Design review of the part built by this model. Coordinates are the model's own, in mm. Round coordinates to 2 decimals unless told otherwise and drop trailing zeros. Order: outer loops, then holes, each group sorted by start corner. A loop starts at its lowest first (then second) coordinate and runs counter-clockwise, first axis right, second up. Notation, with made-up numbers: M 70,-11 L 115,-11 A24 cw 115,24 Z; hole C 54,15 d3. An arc over 180 degrees is marked long. Use a Markdown table: item, result. Add a question column.
(1) The part is to be moulded in two halves that separate along Z. For faces 1 (the face through (434.95, 2.03, -85.78)), 2 (the face through (222, 4, -127)), say which applies: released by +Z, released by -Z, zero draft, split by the parting line, or undercut.
(2) To check wall thickness, follow probe 1 along X at (y, z) = (1.4, -190); probe 2 along X at (y, z) = (3.6, -114.5); probe 3 along X at (y, z) = (2.45, -197.5). State the ranges of each line that lie inside material, in increasing order. Write a range as from..to.
(3) Take a section at D-D (z = -211.5). Write out the cut boundary in (x, y).
(4) Take a section at B-B (z = -65). Write out the cut boundary in (x, y), then the cut area to 3 significant figures.
(5) Take a section at C-C (x = 429). Write out the cut boundary in (y, z).
(6) For pin 1 (0.6 mm diameter, centred on y = 2, z = -114.5, fed in from -X); pin 2 (7 mm diameter, centred on x = 429, z = -65, fed in from -Y), all flat-tipped, find the tip position at first contact; note any pin that passes through.
(7) Take a section at A-A (x = 363). Write out the cut boundary in (y, z).
```python
from build123d import *

# Parameters (mm, degrees)
SKETCH_1_W          = 450
SKETCH_1_H          = 250
EXTRUDE_1_DEPTH     = 4
SKETCH_2_R          = 30
CUT_EXTRUDE_1_DEPTH = 515.797047389
SKETCH_3_R          = 6
SKETCH_3_W          = 20
SKETCH_3_H          = 2
CUT_EXTRUDE_2_DEPTH = 515.797047389


with BuildPart() as part:
    # 草圖1 → 填料-伸長1 (new body)
    with BuildSketch(Plane(origin=(0, 0, 0), x_dir=(1, 0, 0), z_dir=(0, 1, 0))):
        with Locations((225, 125)):
            Rectangle(SKETCH_1_W, SKETCH_1_H)
    extrude(amount=EXTRUDE_1_DEPTH)

    # 草圖2 → 除料-伸長1 (cut, through all)
    with BuildSketch(Plane(origin=(0, 4, 0), x_dir=(1, 0, 0), z_dir=(0, 1, 0))):
        with Locations(Location((78, 190, 0), (0, 0, 270))):
            Circle(SKETCH_2_R)
        with Locations(Location((363, 190, 0), (0, 0, 270))):
            Circle(SKETCH_2_R)
    extrude(amount=-CUT_EXTRUDE_1_DEPTH, mode=Mode.SUBTRACT)

    # 草圖3 → 除料-伸長2 (cut, through all)
    with BuildSketch(Plane(origin=(0, 4, 0), x_dir=(1, 0, 0), z_dir=(0, 1, 0))):
        with Locations(Location((429, 85, 0), (0, 0, 270))):
            Circle(SKETCH_3_R)
        with Locations(Location((429, 65, 0), (0, 0, 270))):
            Circle(SKETCH_3_R)
        with Locations((71.17, 122)):
            Rectangle(SKETCH_3_W, SKETCH_3_H)
        with Locations((71.17, 101)):
            Rectangle(SKETCH_3_W, SKETCH_3_H)
        with Locations((71.17, 115)):
            Rectangle(SKETCH_3_W, SKETCH_3_H)
        with Locations((71.17, 108)):
            Rectangle(SKETCH_3_W, SKETCH_3_H)
        with Locations((71.17, 94)):
            Rectangle(SKETCH_3_W, SKETCH_3_H)
        with Locations((71.17, 87)):
            Rectangle(SKETCH_3_W, SKETCH_3_H)
        with Locations((71.17, 80)):
            Rectangle(SKETCH_3_W, SKETCH_3_H)
    extrude(amount=-CUT_EXTRUDE_2_DEPTH, mode=Mode.SUBTRACT)


solid = part.part
```
Verdict:
| question | item | result |
|---|---|---|
| 1 | face 1 | undercut |
| 1 | face 2 | zero draft |
| 2 | probe 1 | x = 0..48, 108..333, 393..450 |
| 2 | probe 2 | x = 0..61.17, 81.17..450 |
| 2 | probe 3 | x = 0..48.95, 107.05..333.95, 392.05..450 |
| 3 | outline | M 0,0 L 57.08,0 L 57.08,4 L 0,4 Z; M 98.92,0 L 342.08,0 L 342.08,4 L 98.92,4 Z; M 383.92,0 L 450,0 L 450,4 L 383.92,4 Z |
| 4 | outline | M 0,0 L 423,0 L 423,4 L 0,4 Z; M 435,0 L 450,0 L 450,4 L 435,4 Z |
| 4 | area | 1,750 mm^2 |
| 5 | outline | M 0,-250 L 4,-250 L 4,-91 L 0,-91 Z; M 0,-79 L 4,-79 L 4,-71 L 0,-71 Z; M 0,-59 L 4,-59 L 4,0 L 0,0 Z |
| 6 | pin 1 | stops at x = 0 |
| 6 | pin 2 | passes through |
| 7 | outline | M 0,-250 L 4,-250 L 4,-220 L 0,-220 Z; M 0,-160 L 4,-160 L 4,0 L 0,0 Z |
